Can you work these out from the drawing? Everything is in mm from the part's minimum corner. A direction names the side the tool comes from. Give positions to 0.01 mm unless a question says otherwise; leave off trailing zeros. Write each loop counter-clockwise with the first axis right and the second up, starting at its lowest first coordinate (ties: lowest second). Pieces come first, ordered by that corner, then holes. Notation, with made-up numbers: (85.5, 72.25) -> (123.5, 72.25) arc R32 ccw to (123.5, 105.25) -> close; hole circle Ø1 at (38, 75). An arc over 180 degrees is marked (long way). Use one line per item in the form item = value.
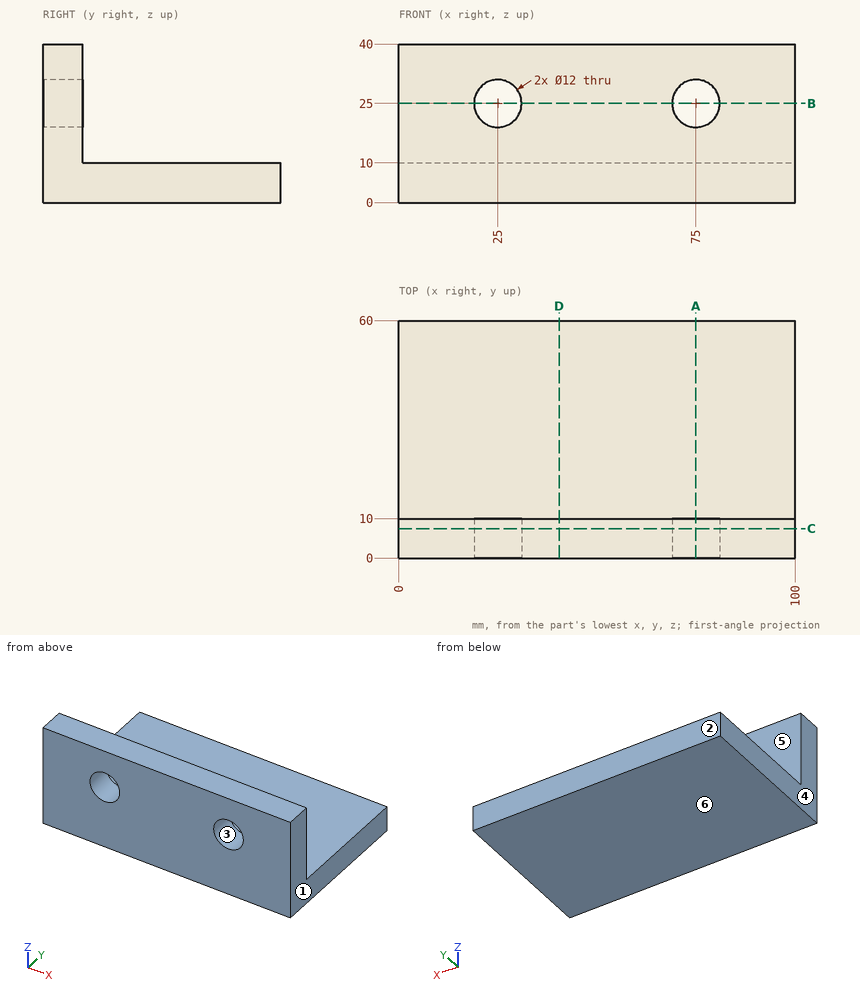
Q1. I want a section at C-C, the plane y = 7.5. Write out the boundary of the cut face in (x, z).
Result set:
outline = (0, 0) -> (100, 0) -> (100, 40) -> (0, 40) -> close; hole circle Ø12 at (25, 25); hole circle Ø12 at (75, 25)
Q2. Which directions (+Z, -Z, +X, -X, +Y, -Y) give clear straight access to the entire face, cutting with the end or side of a thin tool? Please do the marked faces 5 and 6.
Result set:
face_5 = +Z, +X, -X, +Y
face_6 = -Z, +X, -X, +Y, -Y
Q3. Will this pin go through, and if not, where does the flat tip stop? pin 1 Ø6 at (x, z) = (78, 17.5) entering from +Y.
Result set:
pin_1 = 10
Q4. I want a section at D-D, the plane x = 40.5. Write out the boundary of the cut face in (y, z), and give its area (3 significant figures).
Result set:
outline = (0, 0) -> (60, 0) -> (60, 10) -> (10, 10) -> (10, 40) -> (0, 40) -> close
area = 900 mm2
Q5. I want a section at A-A, the plane x = 75. Write out the boundary of the cut face in (y, z).
Result set:
outline = (0, 0) -> (60, 0) -> (60, 10) -> (10, 10) -> (10, 19) -> (0, 19) -> close; (0, 31) -> (10, 31) -> (10, 40) -> (0, 40) -> close
Q6. If we mould it in two halves opening along X, with no side actions, what happens to the marked faces 1, 2, 3 and 4? For each: +X half, -X half, draft (parallel to the pull), parting line (faces both ways), or undercut.
Result set:
face_1 = +X half
face_2 = draft
face_3 = undercut
face_4 = -X half
Q7. If I drill on line 1 along X through (y, z) = (3.5, 25); line 2 along Z through (x, y) = (25, 3); line 3 along Z through (x, y) = (13, 36), over which ranges is the centre line in solid material (lowest first)? Write a range as from..to.
Result set:
line_1 = 0..19, 31..69, 81..100
line_2 = 0..19, 31..40
line_3 = 0..10
Q8. I want a section at B-B, the plane z = 25. Write out the boundary of the cut face in (x, y).
Result set:
outline = (0, 0) -> (19, 0) -> (19, 10) -> (0, 10) -> close; (31, 0) -> (69, 0) -> (69, 10) -> (31, 10) -> close; (81, 0) -> (100, 0) -> (100, 10) -> (81, 10) -> close
